from build123d import *

# Parameters (mm, degrees)
SKETCH1_W           = 27
SKETCH1_H           = 26
BOSS_EXTRUDE1_DEPTH = 15
CUT_EXTRUDE2_DEPTH  = 23.5
SKETCH5_W           = 3.601284645
SKETCH5_H           = 15
CUT_EXTRUDE3_DEPTH  = 33.912763482
SKETCH6_R           = 3
CUT_EXTRUDE4_DEPTH  = 33.912763482
SKETCH7_W           = 5
SKETCH7_H           = 26
BOSS_EXTRUDE2_DEPTH = 20
SKETCH8_W           = 6
SKETCH8_H           = 5.7
BOSS_EXTRUDE3_DEPTH = 3
SKETCH9_W           = 6
SKETCH9_H           = 5.7
BOSS_EXTRUDE4_DEPTH = 3
SKETCH10_R          = 3
CUT_EXTRUDE5_DEPTH  = 42.623463656
SKETCH11_R          = 4.875
CUT_EXTRUDE6_DEPTH  = 31.809901006


with BuildPart() as part:
    # Sketch1 → Boss-Extrude1 (new body)
    with BuildSketch(Plane(origin=(0, 0, 0), x_dir=(1, 0, 0), z_dir=(0, 1, 0))):
        Rectangle(SKETCH1_W, SKETCH1_H)
    extrude(amount=BOSS_EXTRUDE1_DEPTH)

    # Sketch4 → Cut-Extrude2 (cut)
    with BuildSketch(Plane(origin=(13.5, 0, 0), x_dir=(0, 0, -1), z_dir=(1, 0, 0))):
        Polygon((-10, 2), (-7.5, 2), (-7.5, 0), (7.5, 0), (7.5, 2), (10, 2), (10, 8), (7.5, 8), (7.5, 10), (-7.5, 10), (-7.5, 8), (-10, 8), align=None)
    extrude(amount=-CUT_EXTRUDE2_DEPTH, mode=Mode.SUBTRACT)

    # Sketch5 → Cut-Extrude3 (cut, through all)
    with BuildSketch(Plane(origin=(0, 0, -13), x_dir=(-1, 0, 0), z_dir=(0, 0, -1))):
        with Locations((-11.699357678, 7.5)):
            Rectangle(SKETCH5_W, SKETCH5_H)
    extrude(amount=-CUT_EXTRUDE3_DEPTH, mode=Mode.SUBTRACT)

    # Sketch6 → Cut-Extrude4 (cut, through all)
    with BuildSketch(Plane(origin=(0, 0, -13), x_dir=(-1, 0, 0), z_dir=(0, 0, -1))):
        with Locations((0, 5)):
            Circle(SKETCH6_R)
    extrude(amount=-CUT_EXTRUDE4_DEPTH, mode=Mode.SUBTRACT)

    # Sketch7 → Boss-Extrude2 (add)
    with BuildSketch(Plane(origin=(0, 15, 0), x_dir=(1, 0, 0), z_dir=(0, 1, 0))):
        with Locations((-11, 0)):
            Rectangle(SKETCH7_W, SKETCH7_H)
    extrude(amount=BOSS_EXTRUDE2_DEPTH)

    # Sketch8 → Boss-Extrude3 (add)
    with BuildSketch(Plane(origin=(0, 0, -13), x_dir=(-1, 0, 0), z_dir=(0, 0, -1))):
        Polygon((8.5, 35), (-9.898715355, 15), (8.5, 15), align=None)
        with Locations((16.5, 25)):
            Rectangle(SKETCH8_W, SKETCH8_H)
    extrude(amount=-BOSS_EXTRUDE3_DEPTH)

    # Sketch9 → Boss-Extrude4 (add)
    with BuildSketch(Plane.XY.offset(13)):
        Polygon((-8.5, 35), (9.898715355, 15), (-8.5, 15), align=None)
        with Locations((-16.5, 25)):
            Rectangle(SKETCH9_W, SKETCH9_H)
    extrude(amount=-BOSS_EXTRUDE4_DEPTH)

    # Sketch10 → Cut-Extrude5 (cut, through all)
    with BuildSketch(Plane(origin=(-8.5, 0, 0), x_dir=(0, 0, -1), z_dir=(1, 0, 0))):
        with Locations((0, 25)):
            Circle(SKETCH10_R)
    extrude(amount=-CUT_EXTRUDE5_DEPTH, mode=Mode.SUBTRACT)

    # Sketch11 → Cut-Extrude6 (cut, through all)
    with BuildSketch(Plane(origin=(0, 15, 0), x_dir=(1, 0, 0), z_dir=(0, 1, 0))):
        with Locations(Location((0, 0, 0), (0, 0, 270))):
            Circle(SKETCH11_R)
    extrude(amount=-CUT_EXTRUDE6_DEPTH, mode=Mode.SUBTRACT)


solid = part.part
The model under review builds one solid part; all positions refer to its coordinate system, in mm. A direction names the side the tool comes from. Round coordinates to 2 decimals unless told otherwise and drop trailing zeros. Loops run counter-clockwise (first coordinate to the right, second up) from the corner with the lowest first, then second, coordinate; pieces in that order, holes last. Notation, with made-up numbers: M -33.75,-6 L -6.75,-6 A28 ccw -6.75,19 Z; hole C 74.25,87 d8. An arc over 180 degrees is marked long. Answer as CSV lines item,"result". Start each with the question number.
Item 1: Mouldability with a two-part tool opening along Z and no side actions: class faces 1 (the face through (-5, 14, -13)), 2 (the face through (0, 1, -7.5)), 3 (the face through (-19.5, 25, 12)) as released by +Z, released by -Z, zero draft, split by the parting line, or undercut.
Item 2: Wall thickness on line 1 (Y direction, x = -3.75, z = 9.5); line 2 (X direction, y = 5, z = 11.65); line 3 (Y direction, x = -12.2, z = 0): over which ranges is each line inside the solid? List them lowest first. Write a range as [from, to].
Item 3: Consider section D-D (x = -13). Write out the cut boundary in (y, z).
Item 4: Consider section C-C (y = 5). Write out the cut boundary in (x, z), then the cut area to 3 significant figures.
Item 5: Consider section A-A (z = 0). Write out the cut boundary in (x, y) (3 decimals).
Item 6: For faces 4 (the face through (5, 15, 2)), 5 (the face through (0, 8, 9)), 6 (the face through (-16, 25, -10)), 7 (the face through (-17, 27.85, 12)), 8 (the face through (0, 9, 7.5)), list the 3-axis set-ups (+Z, -Z, +X, -X, +Y, -Y) from which the entire face can be reached by the end or side of a thin tool; tool diameter is ignored.
Item 7: Consider section B-B (x = -16.75). Write out the cut boundary in (y, z), then the cut area to 3 significant figures.
Item 8: Insertion check: P1, Ø0.9, axis at x = -18, z = -12, coming from the +Y side; P2, Ø5, axis at x = 3, z = -3.5, coming from the +Y side; P3, Ø7, axis at y = 25, z = 0, coming from the -X side; P4, Ø3.5, axis at x = 0, y = 5, coming from the -Z side. Each pin has a flat end and moves straight along its axis. Give the tip position at first contact, or say it passes through.
Answer:
1,face 1,"released by -Z"
1,face 2,"undercut"
1,face 3,"zero draft"
2,line 1,"y = [0, 2], [8, 15]"
2,line 2,"x = [-13.5, -3], [3, 9.9]"
2,line 3,"y = [0, 22], [28, 35]"
3,outline,"M 0,-13 L 35,-13 L 35,13 L 0,13 Z; hole C 25,0 d6"
4,outline,"M -13.5,-13 L -3,-13 L -3,-10 L -10,-10 L -10,10 L -3,10 L -3,13 L -13.5,13 Z; M 3,-13 L 9.9,-13 L 9.9,-10 L 3,-10 Z; M 3,10 L 9.9,10 L 9.9,13 L 3,13 Z"
4,area,"174 mm^2"
5,outline,"M -13.5,0 L -10,0 L -10,10 L -4.875,10 L -4.875,15 L -8.5,15 L -8.5,22 L -13.5,22 Z; M -13.5,28 L -8.5,28 L -8.5,35 L -13.5,35 Z; M 4.875,10 L 9.899,10 L 9.899,15 L 4.875,15 Z"
6,face 4,"+X, +Y"
6,face 5,"+X"
6,face 6,"-X, +Y, -Y"
6,face 7,"+Z, -Z, -X, +Y"
6,face 8,"+X, -Y"
7,outline,"M 22.15,-13 L 27.85,-13 L 27.85,-10 L 22.15,-10 Z; M 22.15,10 L 27.85,10 L 27.85,13 L 22.15,13 Z"
7,area,"34.2 mm^2"
8,P1,"stops at y = 27.85"
8,P2,"stops at y = 15"
8,P3,"stops at x = -13.5"
8,P4,"passes through"
